from build123d import *

# Parameters (mm, degrees)
SKETCH_1_W      = 2.7
SKETCH_1_H      = 2.2
SKETCH_1_R      = 1.25
SKETCH_1_R_2    = 1.75
EXTRUDE_1_DEPTH = 3


with BuildPart() as part:
    # 草图1 → 凸台-拉伸1 (new body)
    with BuildSketch(Plane(origin=(0, 0, 0), x_dir=(1, 0, 0), z_dir=(0, 1, 0))):
        with BuildLine():
            ThreePointArc((-7, -10.25), (-6.414213562, -11.664213562), (-5, -12.25))
            Line((-5, -12.25), (5, -12.25))
            ThreePointArc((5, -12.25), (6.414213562, -11.664213562), (7, -10.25))
            Line((7, -10.25), (7, 12.25))
            ThreePointArc((7, 12.25), (0, 19.25), (-7, 12.25))
            Line((-7, 12.25), (-7, -10.25))
        make_face()
        with Locations((-3.75, -9.393390946)):
            Rectangle(SKETCH_1_W, SKETCH_1_H, mode=Mode.SUBTRACT)
        with Locations((0, -9.25)):
            Circle(SKETCH_1_R, mode=Mode.SUBTRACT)
        with Locations((3.75, -9.393390946)):
            Rectangle(SKETCH_1_W, SKETCH_1_H, mode=Mode.SUBTRACT)
        with Locations((0, 12.25)):
            Circle(SKETCH_1_R_2, mode=Mode.SUBTRACT)
    extrude(amount=EXTRUDE_1_DEPTH)


solid = part.part
Read the model definition and answer for the solid it produces. Units are mm, in the model's axes. A direction names the side the tool comes from. Round coordinates to 2 decimals unless told otherwise and drop trailing zeros. Write each loop counter-clockwise with the first axis right and the second up, starting at its lowest first coordinate (ties: lowest second). Pieces come first, ordered by that corner, then holes. Notation, with made-up numbers: M -14.75,59.5 L 18.25,59.5 A17 cw 18.25,86.5 Z; hole C 26,-8 d1. An arc over 180 degrees is marked long. Use a Markdown table: item, result.
1) The part is cut by section A-A (y = 1.2). Write down the section's boundary in (x, z).
Answers follow:
| item | result |
|---|---|
| outline | M -7,-12.25 A7 ccw 7,-12.25 L 7,10.25 A2 ccw 5,12.25 L -5,12.25 A2 ccw -7,10.25 Z; hole M -5.1,8.29 L -2.4,8.29 L -2.4,10.49 L -5.1,10.49 Z; hole C 0,-12.25 d3.5; hole C 0,9.25 d2.5; hole M 2.4,8.29 L 5.1,8.29 L 5.1,10.49 L 2.4,10.49 Z |
2) Flat-ended cylindrical pins translate along their axes: pin 1 (1.3 mm diameter, centred on x = -3.5, y = 1.5, fed in from -Z); pin 2 (1.3 mm diameter, centred on x = 4, y = 1, fed in from -Z); pin 3 (1 mm diameter, centred on x = 4.5, y = 0.5, fed in from -Z). Find the tip coordinate at first contact, or state that the pin passes through.
Answers follow:
| item | result |
|---|---|
| pin 1 | stops at z = -18.64 |
| pin 2 | stops at z = -18.4 |
| pin 3 | stops at z = -17.99 |
3) Straight lines are drawn through the part: line 1 along X through (y, z) = (1.2, 9.25); line 2 along Z through (x, y) = (0, 0.8); line 3 along X through (y, z) = (0.6, 10). For each, find the intervals that lie inside material, in ascending order. Write a range as [from, to].
Answers follow:
| item | result |
|---|---|
| line 1 | x = [-7, -5.1], [-2.4, -1.25], [1.25, 2.4], [5.1, 7] |
| line 2 | z = [-19.25, -14], [-10.5, 8], [10.5, 12.25] |
| line 3 | x = [-7, -5.1], [-2.4, -1], [1, 2.4], [5.1, 7] |
4) A tool of negligible diameter and unlimited length cuts with its end or side. For faces 4 (the flat face through (0, 0, -4)), 5 (the flat face through (5.1, 1, 9)), from which of +Z, -Z, +X, -X, +Y, -Y can it reach the whole face along a straight path? Write none if from no direction.
Answers follow:
| item | result |
|---|---|
| face 4 | +Z, -Z, +X, -X, -Y |
| face 5 | +Y, -Y |
5) The part is cut by section C-C (z = 9.25). Write down the section's boundary in (x, y).
Answers follow:
| item | result |
|---|---|
| outline | M -7,0 L -5.1,0 L -5.1,3 L -7,3 Z; M -2.4,0 L -1.25,0 L -1.25,3 L -2.4,3 Z; M 1.25,0 L 2.4,0 L 2.4,3 L 1.25,3 Z; M 5.1,0 L 7,0 L 7,3 L 5.1,3 Z |
6) The part is cut by section B-B (x = 0). Write down the section's boundary in (y, z).
Answers follow:
| item | result |
|---|---|
| outline | M 0,-19.25 L 3,-19.25 L 3,-14 L 0,-14 Z; M 0,-10.5 L 3,-10.5 L 3,8 L 0,8 Z; M 0,10.5 L 3,10.5 L 3,12.25 L 0,12.25 Z |
7) For a pull along X with two mould halves and no side action, classify faces 1 (the flat face through (0, 1, 12.25)), 2 (the flat face through (-4, 1, 8.293)), 3 (the flat face through (-7, 1, -1)) as pulls with the +X half, pulls with the -X half, needs draft (parallel to the pull), parting line crosses it, or undercut.
Answers follow:
| item | result |
|---|---|
| face 1 | needs draft |
| face 2 | undercut |
| face 3 | pulls with the -X half |
